The listing builds one solid part. Answer for the finished solid, in the listing's coordinates (mm). A direction names the side the tool comes from. Round coordinates to 2 decimals unless told otherwise and drop trailing zeros. Order: outer loops, then holes, each group sorted by start corner. A loop starts at its lowest first (then second) coordinate and runs counter-clockwise, first axis right, second up. Notation, with made-up numbers: (42, 37.25) -> (88, 37.25) arc R25 cw to (88, 64.25) -> close; hole circle Ø4 at (75, 84). An arc over 180 degrees is marked (long way). Answer in a Markdown table with one row per item. Add a question column.
```python
from build123d import *

# Parameters (mm, degrees)
SALIENTE_EXTRUIR3_DEPTH = 10
CROQUIS3_R              = 10
CORTAR_EXTRUIR1_DEPTH   = 10
REDONDEO2_R             = 12
CROQUIS4_R              = 1.5
CORTAR_EXTRUIR2_DEPTH   = 45.733638102
REDONDEO3_R             = 3


with BuildPart() as part:
    # Croquis1 → Saliente-Extruir3 (new body)
    with BuildSketch(Plane.XY):
        Polygon((0, 29.5), (-24.396106146, -12.755295351), (-31.396106146, -12.755295351), (-31.396106146, -14.755295351), (-25.556921229, -14.755295351), (25.556921229, -14.755295351), (31.396106146, -14.755295351), (31.396106146, -12.755295351), (24.396106146, -12.755295351), align=None)
    extrude(amount=SALIENTE_EXTRUIR3_DEPTH)

    # Croquis3 → Cortar-Extruir1 (cut)
    with BuildSketch(Plane(origin=(0, 0, 0), x_dir=(-1, 0, 0), z_dir=(0, 0, -1))):
        Circle(CROQUIS3_R)
    extrude(amount=-CORTAR_EXTRUIR1_DEPTH, mode=Mode.SUBTRACT)

    # Redondeo2
    redondeo2_edges = [part.edges().sort_by_distance(p)[0] for p in [
        (0, 29.5, 5),
    ]]
    fillet(redondeo2_edges, radius=REDONDEO2_R)

    # Croquis4 → Cortar-Extruir2 (cut, through all)
    with BuildSketch(Plane(origin=(0, -12.755295351, 0), x_dir=(1, 0, 0), z_dir=(0, 1, 0))):
        with Locations(Location((27.896106146, -5, 0), (0, 0, 180))):
            Circle(CROQUIS4_R)
        with Locations(Location((-27.896106146, -5, 0), (0, 0, 180))):
            Circle(CROQUIS4_R)
    extrude(amount=-CORTAR_EXTRUIR2_DEPTH, mode=Mode.SUBTRACT)

    # Redondeo3
    redondeo3_edges = [part.edges().sort_by_distance(p)[0] for p in [
        (-31.396106146, -13.755295351, 10),
        (-31.396106146, -13.755295351, 0),
        (31.396106146, -13.755295351, 10),
        (31.396106146, -13.755295351, 0),
    ]]
    fillet(redondeo3_edges, radius=REDONDEO3_R)


solid = part.part
```
1. The part is cut by section B-B (x = 0). Give the vertices of the cut face in (y, z), then the cut area to 3 significant figures.
2. The part is cut by section D-D (x = 25.5). Give the vertices of the cut face in (y, z).
3. Straight lines are drawn through the part: line 1 along X through (y, z) = (3.5, 8); line 2 along X through (y, z) = (-5, 4); line 3 along Y through (x, z) = (1, 4). For each, find the intervals that lie inside material, in ascending order.
4. Each of these flat-tipped pins is pushed along its axis until it touches: pin 1 (1 mm diameter, centred on y = -11, z = 7.5, fed in from +X); pin 2 (18 mm diameter, centred on x = 0, y = 0, fed in from -Z); pin 3 (1.5 mm diameter, centred on y = 11.5, z = 8.5, fed in from +X); pin 4 (3.5 mm diameter, centred on x = 26.5, z = 3.5, fed in from +Y). Where does it stop, or does it pass through?
5. The part is cut by section C-C (y = 2.5). Give the vertices of the cut face in (x, z).
6. The mould has two halves that part along X. Classify faces 1 (the flat face through (-31.396, -14, 5)), 2 (the cylindrical face through (-26.4, -13.7, 5.1)), 3 (the cylindrical face through (30.494, -13.741, 0.855)): released by +X, released by -X, zero draft, split by the parting line, or undercut.
7. For faces 4 (the flat face through (26, -12.755, 5)), 5 (the flat face through (-26, -12.755, 5)), 6 (the flat face through (31.396, -14, 5)), determine the directions among +Z, -Z, +X, -X, +Y, -Y from which every point of the face is accessible in a straight line to the end or side of a thin tool.
8. The part is cut by section A-A (z = 5). Give the vertices of the cut face in (x, y), then the cut area to 3 significant figures.
Report:
| question | item | result |
|---|---|---|
| 1 | outline | (-14.76, 0) -> (-10, 0) -> (-10, 10) -> (-14.76, 10) -> close; (10, 0) -> (17.5, 0) -> (17.5, 10) -> (10, 10) -> close |
| 1 | area | 123 mm^2 |
| 2 | outline | (-14.76, 0) -> (-12.76, 0) -> (-12.76, 10) -> (-14.76, 10) -> close |
| 3 | line 1 | x = -15.01 to -9.37, 9.37 to 15.01 |
| 3 | line 2 | x = -19.92 to -8.66, 8.66 to 19.92 |
| 3 | line 3 | y = -14.76 to -9.95, 9.95 to 17.46 |
| 4 | pin 1 | stops at x = 23.67 |
| 4 | pin 2 | passes through |
| 4 | pin 3 | stops at x = 10.83 |
| 4 | pin 4 | stops at y = -12.76 |
| 5 | outline | (-15.59, 0) -> (-9.68, 0) -> (-9.68, 10) -> (-15.59, 10) -> close; (9.68, 0) -> (15.59, 0) -> (15.59, 10) -> (9.68, 10) -> close |
| 6 | face 1 | released by -X |
| 6 | face 2 | undercut |
| 6 | face 3 | released by +X |
| 7 | face 4 | +Z, -Z, +X, +Y |
| 7 | face 5 | +Z, -Z, -X, +Y |
| 7 | face 6 | +Z, -Z, +X, +Y, -Y |
| 8 | outline | (-31.4, -14.76) -> (-29.4, -14.76) -> (-29.4, -12.76) -> (-31.4, -12.76) -> close; (-26.4, -14.76) -> (26.4, -14.76) -> (26.4, -12.76) -> (24.4, -12.76) -> (10.39, 11.5) arc R12 ccw to (-10.39, 11.5) -> (-24.4, -12.76) -> (-26.4, -12.76) -> close; (29.4, -14.76) -> (31.4, -14.76) -> (31.4, -12.76) -> (29.4, -12.76) -> close; hole circle Ø20 at (0, 0) |
| 8 | area | 732 mm^2 |
